Part model, mm, in its own coordinate system. Face numbers are marked on the shaded views. A direction names the side the tool comes from. Coordinates: 2 decimals unless noted, no trailing zeros. Loops run counter-clockwise (first coordinate to the right, second up) from the corner with the lowest first, then second, coordinate; pieces in that order, holes last. Notation, with made-up numbers: M 83,6 L 133,6 A19 cw 133,28 Z; hole C 14,-21.75 d9. An arc over 180 degrees is marked long. Answer as CSV lines item,"result". Start each with the question number.
from build123d import *

# Parameters (mm, degrees)
F0_R     = 1.5
F1_DEPTH = 3
F2_W     = 55
F2_H     = 3
F3_DEPTH = 25
F4_R     = 3
F5_R     = 3
F6_DEPTH = 163.1321276775


with BuildPart() as f1:
    # F0 (on Front) → F1 (new body)
    with BuildSketch(Plane.XZ):
        with BuildLine():
            Line((454.8277321524, 574.7700988736), (454.8277321524, 576.6820907487))
            Line((454.8277321524, 576.6820907487), (420.231500864, 416.5509630712))
            Line((420.231500864, 416.5509630712), (495.9500458773, 416.5509630712))
            Line((495.9500458773, 416.5509630712), (525.231500864, 416.5509630712))
            Line((525.231500864, 416.5509630712), (490.6352695757, 576.6820907487))
            Line((490.6352695757, 576.6820907487), (490.6352695757, 574.7700988736))
            ThreePointArc((490.6352695757, 574.7700988736), (472.731500864, 556.866330162), (454.8277321524, 574.7700988736))
        make_face()
        with Locations((472.731500864, 449.0509630712)):
            Circle(F0_R, mode=Mode.SUBTRACT)
    extrude(amount=F1_DEPTH)

    # F2 (on face) → F3 (join)
    with BuildSketch(Plane.XZ.offset(3)):
        with Locations((472.731500864, 415.0509630712)):
            Rectangle(F2_W, F2_H)
    extrude(amount=-F3_DEPTH)

    # F4
    f4_edges = [f1.edges().sort_by_distance(p)[0] for p in [
        (472.731501, -3, 413.550963),
        (472.731501, 0, 416.550963),
    ]]
    fillet(f4_edges, radius=F4_R)

    # F5 (on face) → F6 (cut, through all)
    with BuildSketch(Plane(origin=(0, 0, 413.5509630712), x_dir=(1, 0, 0), z_dir=(0, 0, -1))):
        with Locations((472.731500864, -6.5)):
            Circle(F5_R)
    extrude(amount=-F6_DEPTH, mode=Mode.SUBTRACT)


solid = f1.part
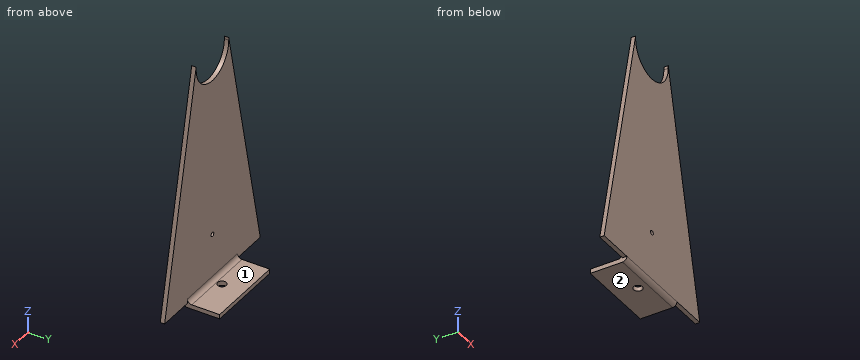
Q1. Slice it at D-D, the plane z = 460. Write the cut outline in (x, y).
Q2. Slice it at C-C, the plane y = 13.5. Write the cut outline in (x, z).
Q3. Slice it at A-A, the plane y = 6.5. Write the cut outline in (x, z).
Q4. Slice it at B-B, the plane x = 495. Write the cut outline in (y, z), and give its area (3 significant figures).
Q5. Wall check: L1, parallel to X at y = 6.5, z = 414.9; L2, parallel to Y at x = 458, z = 558; L3, parallel to Z at x = 487.5, y = 7. Give the ranges that are in metal, low to high.
Q6. Flat gauge pins, fed straight in: P1, Ø3, axis at x = 481, y = 5.5, coming from the +Z side; P2, Ø6, axis at x = 511.5, z = 495.5, coming from the +Y side; P3, Ø5, axis at x = 486, z = 458.5, coming from the +Y side; P4, Ø3.5, axis at x = 435.5, y = -2, coming from the -Z side. Where does each tip first touch, or does it go through?
Q7. Tool access for the marked faces 1 and 2: list every direction of +Z, -Z, +X, -X, +Y, -Y with a clear straight run to the whole face (end or side of a thin tool).
Solved:
1,outline,"M 429.62,-3 L 515.84,-3 L 515.84,0 L 429.62,0 Z"
2,outline,"M 445.23,413.55 L 500.23,413.55 L 500.23,416.55 L 445.23,416.55 Z"
3,outline,"M 445.23,413.55 L 469.73,413.55 L 469.73,416.55 L 445.23,416.55 Z; M 475.73,413.55 L 500.23,413.55 L 500.23,416.55 L 475.73,416.55 Z"
4,outline,"M -3,416.55 A3 ccw 0,413.55 L 22,413.55 L 22,416.55 L 3,416.55 A3 cw 0,419.55 L 0,556.48 L -3,556.48 Z"
4,area,"495 mm2"
5,L1,"x = 445.23 to 469.73, 475.73 to 500.23"
5,L2,"y = -3 to 0"
5,L3,"z = 413.55 to 416.55"
6,P1,"stops at z = 416.55"
6,P2,"passes through"
6,P3,"stops at y = 0"
6,P4,"stops at z = 416.55"
7,face 1,"+Z, +X, -X, +Y"
7,face 2,"-Z, +X, -X, +Y, -Y"
